Check sheet for the modelled part. Datum: model origin and axes. Units: mm. Face numbers are marked on the shaded views. A direction names the side the tool comes from. Round coordinates to 2 decimals unless told otherwise and drop trailing zeros. Order: outer loops, then holes, each group sorted by start corner. A loop starts at its lowest first (then second) coordinate and runs counter-clockwise, first axis right, second up. Notation, with made-up numbers: (14.5, -37) -> (64.5, -37) arc R36 ccw to (64.5, 0) -> close; hole circle Ø11 at (-3, 29). An arc over 180 degrees is marked (long way). Answer in a Markdown table with one row per item. Add a question column.
1. Sectioned sample at D-D, the plane y = 8. Record the boundary of the cut face in (x, z).
2. Draft check along Y on the marked faces 3, 4 and 5. Enter one of: +Y half, -Y half, draft (parallel to the pull), parting line (faces both ways), or undercut.
3. Access from +Z, -Z, +X, -X, +Y, -Y to the whole of each face (thin tool, end or side, straight path). Record for the marked faces 1 and 2.
4. Sectioned sample at B-B, the plane y = 1.25. Record the boundary of the cut face in (x, z), then the cut area to 3 significant figures.
5. Sectioned sample at A-A, the plane x = 0.85. Record the boundary of the cut face in (y, z), then the cut area to 3 significant figures.
6. Depth check by flat-ended pin: P1, Ø0.5, axis at x = 0, y = 4.5, coming from the -Z side. Enter the tip coordinate at first touch or a pass-through.
7. Material ranges on L1, parallel to Y at x = 0, z = -0.1; L2, parallel to Z at x = -0.3, y = 5; L3, parallel to X at y = 1, z = 0.35, recorded low to high. Write a range as from..to.
```python
from build123d import *

# Parameters (mm, degrees)
BOX_W           = 3
BOX_H           = 9
BOX_DEPTH       = 1
SKETCH_R        = 1
POCKET_DEPTH    = 3
BOX001_W        = 2
BOX001_H        = 4
BOX001_DEPTH    = 2
POCKET001_DEPTH = 0.15
FILLET_R        = 1


with BuildPart() as part:
    # Box → Box (join)
    with BuildSketch(Plane(origin=(-1.5, 0, -0.5), x_dir=(1, 0, 0), z_dir=(0, 0, 1))):
        with Locations((1.5, 4.5)):
            Rectangle(BOX_W, BOX_H)
    extrude(amount=BOX_DEPTH)

    # Sketch → Pocket (cut, symmetric)
    with BuildSketch(Plane.XY):
        with Locations((0, 1.5)):
            Circle(SKETCH_R)
    extrude(amount=POCKET_DEPTH, both=True, mode=Mode.SUBTRACT)

    # Sphere → Sphere (revolve, cut)
    with BuildSketch(Plane(origin=(-7, 5, 0), x_dir=(0, 1, 0), z_dir=(0, 0, -1))):
        with BuildLine():
            ThreePointArc((0, -6.5), (6.5, 0), (0, 6.5))
            Line((0, 6.5), (0, -6.5))
        make_face()
    sphere = revolve(axis=Axis((-7, 5, 0), (1, 0, 0)), mode=Mode.SUBTRACT)

    # Mirrored: Sphere across YZ
    add(sphere.mirror(Plane.YZ), mode=Mode.SUBTRACT)

    # Box001 → Box001 (cut)
    with BuildSketch(Plane(origin=(0.5, 5, -1), x_dir=(1, 0, 0), z_dir=(0, 0, 1))):
        with Locations((1, 2)):
            Rectangle(BOX001_W, BOX001_H)
    box001 = extrude(amount=BOX001_DEPTH, mode=Mode.SUBTRACT)

    # Mirrored001: Box001 across YZ
    add(box001.mirror(Plane.YZ), mode=Mode.SUBTRACT)

    # Sketch001 (on Face4 of Mirrored001) → Pocket001 (cut, symmetric)
    with BuildSketch(Plane(origin=(0.5, 5, -0.5), x_dir=(1, 0, 0), z_dir=(0, 0, -1))):
        Polygon((-0.25, -3.9), (-0.75, -3.9), (-1, 2.4), (0, 2.4), align=None)
    extrude(amount=POCKET001_DEPTH, both=True, mode=Mode.SUBTRACT)

    # Fillet
    fillet_edges = [part.edges().sort_by_distance(p)[0] for p in [
        (-1.5, 0, 0),
        (1.5, 0, 0),
    ]]
    fillet(fillet_edges, radius=FILLET_R)


solid = part.part
```
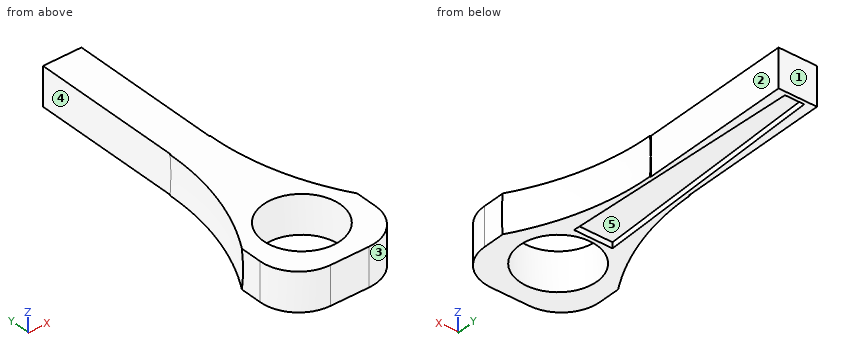
Answer key:
| question | item | result |
|---|---|---|
| 1 | outline | (-0.5, -0.5) -> (-0.29, -0.5) -> (-0.29, -0.35) -> (0.29, -0.35) -> (0.29, -0.5) -> (0.5, -0.5) -> (0.5, 0.5) -> (-0.5, 0.5) -> close |
| 2 | face 3 | -Y half |
| 2 | face 4 | draft |
| 2 | face 5 | undercut |
| 3 | face 1 | +Z, -Z, +X, -X, +Y |
| 3 | face 2 | +Z, -Z, +X, +Y |
| 4 | outline | (-1.5, -0.5) -> (-0.97, -0.5) -> (-0.97, 0.5) -> (-1.5, 0.5) -> close; (0.97, -0.5) -> (1.5, -0.5) -> (1.5, 0.5) -> (0.97, 0.5) -> close |
| 4 | area | 1.06 mm² |
| 5 | outline | (0.06, -0.5) -> (0.97, -0.5) -> (0.97, 0.5) -> (0.06, 0.5) -> close; (2.03, -0.5) -> (2.96, -0.5) arc R2.1 cw to (2.96, 0.5) -> (2.03, 0.5) -> close |
| 5 | area | 1.80 mm² |
| 6 | P1 | stops at z = -0.35 |
| 7 | L1 | y = 0..0.5, 2.5..9 |
| 7 | L2 | z = -0.35..0.5 |
| 7 | L3 | x = -1.5..-0.87, 0.87..1.5 |
